For this review, use the dimensioned drawing (mm, ordinates from the lowest corner) and the shaded views. Coordinates: 2 decimals unless noted, no trailing zeros. Write each loop counter-clockwise with the first axis right and the second up, starting at its lowest first coordinate (ties: lowest second). Pieces come first, ordered by that corner, then holes. Notation, with made-up numbers: (72, 2) -> (82, 2) arc R10 cw to (82, 21) -> close; hole circle Ø10 at (-26, 56.5). An arc over 180 degrees is marked (long way). Put each result on its own line as item: value. Start each with the question number.
Item 1: Consider section A-A on y = 32.5. Give the boundary of the cut face in (x, z).
Item 2: To check wall thickness, follow L1, parallel to Y at x = 37.5, z = 1.1; L2, parallel to X at y = 10, z = 1.35; L3, parallel to Y at x = 43.5, z = 1.7. State the ranges of each line that lie inside material, in increasing order.
Item 3: Consider section B-B on x = 37.5. Give the boundary of the cut face in (y, z), and give its area (3 significant figures).
Item 4: Insertion check: P1, Ø1, axis at x = 55, z = 0.5, coming from the -Y side; P2, Ø0.6, axis at y = 14, z = 0.5, coming from the +X side; P3, Ø1, axis at x = 21, z = 1.5, coming from the +Y side; P4, Ø2, axis at x = 37.5, y = 32.5, coming from the -Z side. Each pin has a flat end and moves straight along its axis. Give the tip position at first contact, or say it passes through.
Item 5: Consider section D-D on y = 82.5. Give the boundary of the cut face in (x, z), and give its area (3 significant figures).
Item 6: Consider section C-C on z = 1.05. Give the boundary of the cut face in (x, y), and give its area (3 significant figures).
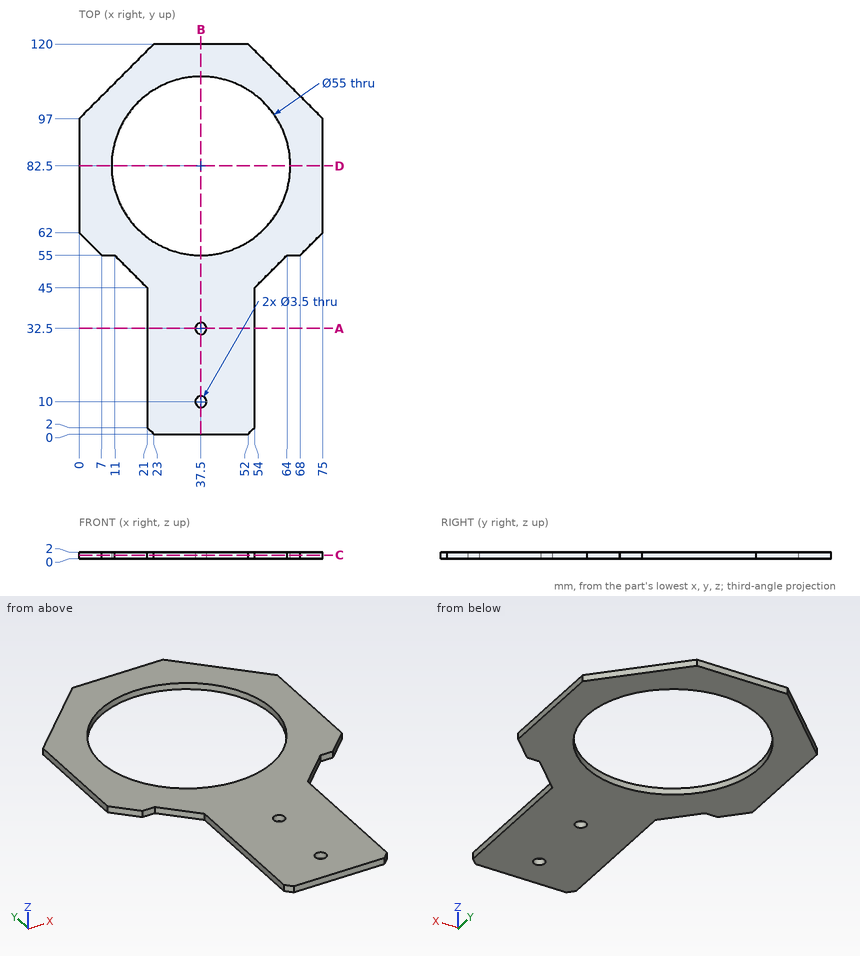
Return value:
1. outline: (21, 0) -> (35.75, 0) -> (35.75, 2) -> (21, 2) -> close; (39.25, 0) -> (54, 0) -> (54, 2) -> (39.25, 2) -> close
2. L1: 0 to 8.25, 11.75 to 30.75, 34.25 to 55, 110 to 120
2. L2: 21 to 35.75, 39.25 to 54
2. L3: 0 to 55.66, 109.34 to 120
3. outline: (0, 0) -> (8.25, 0) -> (8.25, 2) -> (0, 2) -> close; (11.75, 0) -> (30.75, 0) -> (30.75, 2) -> (11.75, 2) -> close; (34.25, 0) -> (55, 0) -> (55, 2) -> (34.25, 2) -> close; (110, 0) -> (120, 0) -> (120, 2) -> (110, 2) -> close
3. area: 116 mm^2
4. P1: y = 45.5
4. P2: x = 54
4. P3: y = 118.5
4. P4: through
5. outline: (0, 0) -> (10, 0) -> (10, 2) -> (0, 2) -> close; (65, 0) -> (75, 0) -> (75, 2) -> (65, 2) -> close
5. area: 40.0 mm^2
6. outline: (0, 62) -> (7, 55) -> (11, 55) -> (21, 45) -> (21, 2) -> (23, 0) -> (52, 0) -> (54, 2) -> (54, 45) -> (64, 55) -> (68, 55) -> (75, 62) -> (75, 97) -> (52, 120) -> (23, 120) -> (0, 97) -> close; hole circle Ø55 at (37.5, 82.5); hole circle Ø3.5 at (37.5, 10); hole circle Ø3.5 at (37.5, 32.5)
6. area: 3,810 mm^2
